from build123d import *
from OCP.BRepFilletAPI import BRepFilletAPI_MakeChamfer

# Parameters (mm, degrees)
SKETCH_1_W          = 405
SKETCH_1_H          = 173
EXTRUDE_1_DEPTH     = 190
SKETCH_2_W          = 405
SKETCH_2_H          = 173
SKETCH_2_W_2        = 400
SKETCH_2_H_2        = 167
CUT_EXTRUDE_1_DEPTH = 9
SKETCH_3_W          = 405
SKETCH_3_H          = 6
CUT_EXTRUDE_2_DEPTH = 1
SKETCH_4_W          = 6
SKETCH_4_H          = 173
CUT_EXTRUDE_3_DEPTH = 1
SKETCH_5_W          = 404
SKETCH_5_H          = 6
CUT_EXTRUDE_4_DEPTH = 1
SKETCH_6_W          = 6
SKETCH_6_H          = 171
CUT_EXTRUDE_5_DEPTH = 1
CHAMFER_1_SIZE      = 6
CHAMFER_1_SIZE_2    = 2
CHAMFER_2_SIZE      = 2
CHAMFER_2_SIZE_2    = 6
SKETCH_7_W          = 64.686
SKETCH_7_H          = 163.6
SKETCH_7_W_2        = 64.682
CUT_EXTRUDE_6_DEPTH = 183


# Some blends are built 0.0001 mm under size
with BuildPart() as part:
    # 草图1 → 凸台-拉伸1 (new body)
    with BuildSketch(Plane.XY):
        with Locations((202.5, 86.5)):
            Rectangle(SKETCH_1_W, SKETCH_1_H)
    extrude(amount=EXTRUDE_1_DEPTH)

    # 草图2 → 切除-拉伸1 (cut)
    with BuildSketch(Plane(origin=(0, 0, 0), x_dir=(-1, 0, 0), z_dir=(0, 0, -1))):
        with Locations((-202.5, 86.5)):
            Rectangle(SKETCH_2_W, SKETCH_2_H)
        with Locations((-202.5, 86.5)):
            Rectangle(SKETCH_2_W_2, SKETCH_2_H_2, mode=Mode.SUBTRACT)
    extrude(amount=-CUT_EXTRUDE_1_DEPTH, mode=Mode.SUBTRACT)

    # 草图3 → 切除-拉伸2 (cut)
    with BuildSketch(Plane.XZ):
        with Locations((202.5, 12)):
            Rectangle(SKETCH_3_W, SKETCH_3_H)
    extrude(amount=-CUT_EXTRUDE_2_DEPTH, mode=Mode.SUBTRACT)

    # 草图4 → 切除-拉伸3 (cut)
    with BuildSketch(Plane(origin=(405, 0, 0), x_dir=(0, 0, -1), z_dir=(1, 0, 0))):
        with Locations((-12, 86.5)):
            Rectangle(SKETCH_4_W, SKETCH_4_H)
    extrude(amount=-CUT_EXTRUDE_3_DEPTH, mode=Mode.SUBTRACT)

    # 草图5 → 切除-拉伸4 (cut)
    with BuildSketch(Plane(origin=(0, 173, 0), x_dir=(1, 0, 0), z_dir=(0, 1, 0))):
        with Locations((202, -12)):
            Rectangle(SKETCH_5_W, SKETCH_5_H)
    extrude(amount=-CUT_EXTRUDE_4_DEPTH, mode=Mode.SUBTRACT)

    # 草图6 → 切除-拉伸5 (cut)
    with BuildSketch(Plane.ZY):
        with Locations((12, 86.5)):
            Rectangle(SKETCH_6_W, SKETCH_6_H)
    extrude(amount=-CUT_EXTRUDE_5_DEPTH, mode=Mode.SUBTRACT)

    # 倒角1
    # the kernel refuses this chamfer: 6, 2 mm, written as the material it takes off along each edge
    with BuildSketch(Plane(origin=(1, -14.570366064, 9), x_dir=(-0.012185754582199162, 0, 0.9999257509361694), z_dir=(0, 1, 0))) as chamfer_1_piece_1_section:
        Polygon((CHAMFER_1_SIZE * 0.999925750936, CHAMFER_1_SIZE * 0.0121857545822), (-CHAMFER_1_SIZE_2 * 0.0121857545822, CHAMFER_1_SIZE_2 * 0.999925750936), (0, 0), align=None)
    chamfer_1_piece_1 = extrude(amount=202.140732128, mode=Mode.PRIVATE)
    chamfer_1_piece_1 = split(chamfer_1_piece_1, bisect_by=Plane(origin=(2.5, 2, 11.1), z_dir=(-1, 0, 0)), keep=Keep.TOP, mode=Mode.PRIVATE)
    add(chamfer_1_piece_1, mode=Mode.SUBTRACT)
    with BuildSketch(Plane(origin=(1, -14.570366064, 9), x_dir=(-0.012185754582199162, 0, 0.9999257509361694), z_dir=(0, 1, 0))) as chamfer_1_piece_2_section:
        Polygon((CHAMFER_1_SIZE * 0.999925750936, CHAMFER_1_SIZE * 0.0121857545822), (-CHAMFER_1_SIZE_2 * 0.0121857545822, CHAMFER_1_SIZE_2 * 0.999925750936), (0, 0), align=None)
    chamfer_1_piece_2 = extrude(amount=202.140732128, mode=Mode.PRIVATE)
    chamfer_1_piece_2 = split(chamfer_1_piece_2, bisect_by=Plane(origin=(2.666666667, 3, 9.5), z_dir=(0, -1, 0)), keep=Keep.TOP, mode=Mode.PRIVATE)
    add(chamfer_1_piece_2, mode=Mode.SUBTRACT)
    with BuildSketch(Plane(origin=(1, -14.570366064, 9), x_dir=(-0.012185754582199162, 0, 0.9999257509361694), z_dir=(0, 1, 0))) as chamfer_1_piece_3_section:
        Polygon((CHAMFER_1_SIZE * 0.999925750936, CHAMFER_1_SIZE * 0.0121857545822), (-CHAMFER_1_SIZE_2 * 0.0121857545822, CHAMFER_1_SIZE_2 * 0.999925750936), (0, 0), align=None)
    chamfer_1_piece_3 = extrude(amount=202.140732128, mode=Mode.PRIVATE)
    chamfer_1_piece_3 = split(chamfer_1_piece_3, bisect_by=Plane(origin=(2.666666667, 170, 9.5), z_dir=(0, 1, 0)), keep=Keep.TOP, mode=Mode.PRIVATE)
    add(chamfer_1_piece_3, mode=Mode.SUBTRACT)
    with BuildSketch(Plane(origin=(404, -14.570366064, 9), x_dir=(-0.9940388851139268, 0, -0.10902612017980623), z_dir=(0, 1, 0))) as chamfer_1_piece_4_section:
        Polygon((CHAMFER_1_SIZE_2 * 0.994038885114, CHAMFER_1_SIZE_2 * 0.10902612018), (-CHAMFER_1_SIZE * 0.10902612018, CHAMFER_1_SIZE * 0.994038885114), (0, 0), align=None)
    chamfer_1_piece_4 = extrude(amount=202.140732128, mode=Mode.PRIVATE)
    chamfer_1_piece_4 = split(chamfer_1_piece_4, bisect_by=Plane(origin=(402.333333333, 3, 9.5), z_dir=(0, -1, 0)), keep=Keep.TOP, mode=Mode.PRIVATE)
    add(chamfer_1_piece_4, mode=Mode.SUBTRACT)
    with BuildSketch(Plane(origin=(404, -14.570366064, 9), x_dir=(-0.9940388851139268, 0, -0.10902612017980623), z_dir=(0, 1, 0))) as chamfer_1_piece_5_section:
        Polygon((CHAMFER_1_SIZE_2 * 0.994038885114, CHAMFER_1_SIZE_2 * 0.10902612018), (-CHAMFER_1_SIZE * 0.10902612018, CHAMFER_1_SIZE * 0.994038885114), (0, 0), align=None)
    chamfer_1_piece_5 = extrude(amount=202.140732128, mode=Mode.PRIVATE)
    chamfer_1_piece_5 = split(chamfer_1_piece_5, bisect_by=Plane(origin=(402.5, 86.5, 11.1), z_dir=(1, 0, 0)), keep=Keep.TOP, mode=Mode.PRIVATE)
    add(chamfer_1_piece_5, mode=Mode.SUBTRACT)
    with BuildSketch(Plane(origin=(404, -14.570366064, 9), x_dir=(-0.9940388851139268, 0, -0.10902612017980623), z_dir=(0, 1, 0))) as chamfer_1_piece_6_section:
        Polygon((CHAMFER_1_SIZE_2 * 0.994038885114, CHAMFER_1_SIZE_2 * 0.10902612018), (-CHAMFER_1_SIZE * 0.10902612018, CHAMFER_1_SIZE * 0.994038885114), (0, 0), align=None)
    chamfer_1_piece_6 = extrude(amount=202.140732128, mode=Mode.PRIVATE)
    chamfer_1_piece_6 = split(chamfer_1_piece_6, bisect_by=Plane(origin=(402.333333333, 170, 9.5), z_dir=(0, 1, 0)), keep=Keep.TOP, mode=Mode.PRIVATE)
    add(chamfer_1_piece_6, mode=Mode.SUBTRACT)

    # 倒角2
    chamfer_2_edges_1 = [part.edges().sort_by_distance(p)[0] for p in [
        (202.5, 172, 9),
    ]]
    chamfer_2_side_1 = [part.faces().sort_by_distance(p)[0] for p in [
        (202.5, 171.96, 9),
    ]]
    chamfer_2_edges_2 = [part.edges().sort_by_distance(p)[0] for p in [
        (202.5, 1, 9),
    ]]
    chamfer_2_side_2 = [part.faces().sort_by_distance(p)[0] for p in [
        (202.5, 1.04, 9),
    ]]
    chamfer_2 = BRepFilletAPI_MakeChamfer(part.part.solid().wrapped)
    for e in chamfer_2_edges_1:
        chamfer_2.Add(CHAMFER_2_SIZE - 0.0001, CHAMFER_2_SIZE_2 - 0.0001, e.wrapped, chamfer_2_side_1[0].wrapped)
    for e in chamfer_2_edges_2:
        chamfer_2.Add(CHAMFER_2_SIZE - 0.0001, CHAMFER_2_SIZE_2 - 0.0001, e.wrapped, chamfer_2_side_2[0].wrapped)
    add(Compound.cast(chamfer_2.Shape()), mode=Mode.REPLACE)  # a hair under: the kernel refuses the full size

    # 草图7 → 切除-拉伸6 (cut)
    with BuildSketch(Plane(origin=(0, 0, 0), x_dir=(-1, 0, 0), z_dir=(0, 0, -1))):
        with Locations((-235.693, 86.5)):
            Rectangle(SKETCH_7_W, SKETCH_7_H)
        with Locations((-169.307, 86.5)):
            Rectangle(SKETCH_7_W, SKETCH_7_H)
        with Locations((-102.923, 86.5)):
            Rectangle(SKETCH_7_W_2, SKETCH_7_H)
        with Locations((-36.541, 86.5)):
            Rectangle(SKETCH_7_W_2, SKETCH_7_H)
        with Locations((-302.077, 86.5)):
            Rectangle(SKETCH_7_W_2, SKETCH_7_H)
        with Locations((-368.459, 86.5)):
            Rectangle(SKETCH_7_W_2, SKETCH_7_H)
    extrude(amount=-CUT_EXTRUDE_6_DEPTH, mode=Mode.SUBTRACT)


solid = part.part
Work out the finished part from the listing and answer in its coordinate system (mm). A direction names the side the tool comes from. Round coordinates to 2 decimals unless told otherwise and drop trailing zeros. Write each loop counter-clockwise with the first axis right and the second up, starting at its lowest first coordinate (ties: lowest second). Pieces come first, ordered by that corner, then holes.
1) Straight lines are drawn through the part: line 1 (Y direction, x = 337, z = 58); line 2 (Y direction, x = 244, z = 9); line 3 (Z direction, x = 320, y = 73). For each, find the intervals that lie inside material, in ascending order.
2) A cutting plane is placed at A-A (z = 96.5). Give the vertices of the cut face in (x, y), plus the area to 3 significant figures.
3) Given pin 1 Ø5 at (y, z) = (82.5, 4) entering from +X; pin 2 Ø5 at (x, z) = (291.5, 7) entering from +Y; pin 3 Ø4 at (x, y) = (88.5, 153) entering from -Z, each flat-ended and moving along its own axis, determine where each tip first touches the part or whether it passes through.
4) The mould has two halves that part along X. Classify faces 4 (the flat face through (103, 88, 183)), 5 (the flat face through (402.5, 85, 5)), 6 (the flat face through (200, 88, 190)): pulls with the +X half, pulls with the -X half, needs draft (parallel to the pull), parting line crosses it, or undercut.
5) A tool of negligible diameter and unlimited length cuts with its end or side. For faces 1 (the flat face through (2.5, 85, 5)), 2 (the flat face through (205, 3, 5)), 3 (the flat face through (369, 168.3, 90)), from which of +Z, -Z, +X, -X, +Y, -Y can it reach the whole face along a straight path? Write none if from no direction.
Completed:
1. line 1: y = 0 to 4.7, 168.3 to 173
1. line 2: y = 3 to 4.7, 168.3 to 170
1. line 3: z = 183 to 190
2. outline: (0, 0) - (405, 0) - (405, 173) - (0, 173) - close; hole (4.2, 4.7) - (68.88, 4.7) - (68.88, 168.3) - (4.2, 168.3) - close; hole (70.58, 4.7) - (135.26, 4.7) - (135.26, 168.3) - (70.58, 168.3) - close; hole (136.96, 4.7) - (201.65, 4.7) - (201.65, 168.3) - (136.96, 168.3) - close; hole (203.35, 4.7) - (268.04, 4.7) - (268.04, 168.3) - (203.35, 168.3) - close; hole (269.74, 4.7) - (334.42, 4.7) - (334.42, 168.3) - (269.74, 168.3) - close; hole (336.12, 4.7) - (400.8, 4.7) - (400.8, 168.3) - (336.12, 168.3) - close
2. area: 6,570 mm2
3. pin 1: stops at x = 402.5
3. pin 2: stops at y = 170.17
3. pin 3: stops at z = 183
4. face 4: undercut
4. face 5: pulls with the +X half
4. face 6: needs draft
5. face 1: -Z, -X, +Y, -Y
5. face 2: -Z, +X, -X, -Y
5. face 3: -Z
